from build123d import *

# Parameters (mm, degrees)
F1_DEPTH  = 31.75
F2_W      = 25.4
F2_H      = 25.4
F3_DEPTH  = 10
F4_R      = 5
F6_D      = 5.5
F8_D      = 4.2
F11_DEPTH = 5


with BuildPart() as f1:
    # F0 (on Top) → F1 (new body)
    with BuildSketch(Plane.XY):
        with BuildLine():
            Line((0, 48), (0, 0))
            Line((0, 0), (66.3673695676, 0))
            Line((66.3673695676, 0), (66.3673695676, 19.4482603496))
            ThreePointArc((66.3673695676, 19.4482603496), (67.5014803837, 21.6950829682), (69.85, 22.6))
            Line((69.85, 22.6), (100, 22.6))
            Line((100, 22.6), (100, 48))
            Line((100, 48), (0, 48))
        make_face()
    extrude(amount=F1_DEPTH)

    # F2 (on face) → F3 (cut)
    with BuildSketch(Plane(origin=(0, 0, 0), x_dir=(1, 0, 0), z_dir=(0, 0, -1))):
        with Locations((34.925, -35.3)):
            Rectangle(F2_W, F2_H)
    extrude(amount=-F3_DEPTH, mode=Mode.SUBTRACT)

    # F4
    f4_edges = [f1.edges().sort_by_distance(p)[0] for p in [
        (22.225, 22.6, 5),
        (47.625, 22.6, 5),
    ]]
    fillet(f4_edges, radius=F4_R)

    # F6 (through all)
    with Locations(Plane.XY.offset(31.75)):
        with Locations((14.1336847838, 11.3), (52.2336847838, 11.3)):
            Hole(F6_D / 2)

    # F8 (through all)
    with Locations(Plane.XY.offset(31.75)):
        with Locations((87.3, 35.3)):
            Hole(F8_D / 2)

    # F10 (on face) → F11 (cut)
    with BuildSketch(Plane(origin=(0, 0, 0), x_dir=(1, 0, 0), z_dir=(0, 0, -1))):
        with BuildLine():
            Line((17.225, -27.6), (17.225, -48))
            Line((17.225, -48), (52.625, -48))
            Line((52.625, -48), (52.625, -27.6))
            ThreePointArc((52.625, -27.6), (51.1605339059, -24.0644660941), (47.625, -22.6))
            Line((47.625, -22.6), (22.225, -22.6))
            ThreePointArc((22.225, -22.6), (18.6894660941, -24.0644660941), (17.225, -27.6))
        make_face()
    extrude(amount=-F11_DEPTH, mode=Mode.SUBTRACT)


solid = f1.part
Model file for the job. Use its own axes, mm. A direction names the side the tool comes from. Round coordinates to 2 decimals unless told otherwise and drop trailing zeros. Order: outer loops, then holes, each group sorted by start corner. A loop starts at its lowest first (then second) coordinate and runs counter-clockwise, first axis right, second up. Notation, with made-up numbers: M -36,82 L 14,82 A19 cw 14,94 Z; hole C -4,-13.5 d3. An arc over 180 degrees is marked long. Write each question's results on one line, items separated by ' | '. Start each with the question number.
(1) Saw through at B-B, the plane x = 87.3. Give the cut face in (y, z).
(2) Saw through at D-D, the plane z = 26. Give the cut face in (x, y), then the cut area to 3 significant figures.
(3) Probe probe 1 along Y at (x, z) = (87, 20); probe 2 along X at (y, z) = (44.5, 7.5) (3 decimals); probe 3 along Y at (x, z) = (85, 3.5). List the from-to ranges inside material, lowest first. Write a range as from..to.
(4) Which spindle directions (+Z, -Z, +X, -X, +Y, -Y) get a long thin tool onto all of the face, cutting with end or side? Do faces 1 (the face through (85, 22.6, 16)), 2 (the face through (16.32, 9.63, 15.65)), 3 (the face through (23.651, 24.104, 7.535)). Say none if no direction does.
(5) Drop flat-ended pins along their axis: pin 1 (9.5 mm diameter, centred on y = 5.5, z = 21, fed in from +X); pin 2 (11 mm diameter, centred on x = 47, y = 30, fed in from -Z); pin 3 (1.5 mm diameter, centred on x = 10.5, z = 4, fed in from -Y); pin 4 (3 mm diameter, centred on x = 30.5, z = 3.5, fed in from +Y). Give the stop position or say it passes through.
(6) Two-plate mould, pull along X, no slides. Class faces 4 (the face through (22.225, 38, 7)), 5 (the face through (0, 24, 16)), 6 (the face through (38, 24, 31.75)): pulls with the +X half, pulls with the -X half, needs draft (parallel to the pull), parting line crosses it, or undercut.
(7) Saw through at A-A, the plane y = 11.3. Give the cut face in (x, z).
(8) Saw through at C-C, the plane y = 35.3. Give the cut face in (x, z) (3 decimals).
Established:
1) outline: M 22.6,0 L 33.2,0 L 33.2,31.75 L 22.6,31.75 Z; M 37.4,0 L 48,0 L 48,31.75 L 37.4,31.75 Z
2) outline: M 0,0 L 66.37,0 L 66.37,19.45 A3.5 cw 69.85,22.6 L 100,22.6 L 100,48 L 0,48 Z; hole C 14.13,11.3 d5.5; hole C 52.23,11.3 d5.5; hole C 87.3,35.3 d4.2 | area: 3,980 mm^2
3) probe 1: y = 22.6..33.22, 37.38..48 | probe 2: x = 0..22.225, 47.625..100 | probe 3: y = 22.6..48
4) face 1: +Z, -Z, +X, -Y | face 2: +Z, -Z | face 3: -Z, +Y
5) pin 1: stops at x = 66.37 | pin 2: stops at z = 5 | pin 3: stops at y = 0 | pin 4: stops at y = 22.6
6) face 4: undercut | face 5: pulls with the -X half | face 6: needs draft
7) outline: M 0,0 L 11.38,0 L 11.38,31.75 L 0,31.75 Z; M 16.88,0 L 49.48,0 L 49.48,31.75 L 16.88,31.75 Z; M 54.98,0 L 66.37,0 L 66.37,31.75 L 54.98,31.75 Z
8) outline: M 0,0 L 17.225,0 L 17.225,5 L 22.225,5 L 22.225,10 L 47.625,10 L 47.625,5 L 52.625,5 L 52.625,0 L 85.2,0 L 85.2,31.75 L 0,31.75 Z; M 89.4,0 L 100,0 L 100,31.75 L 89.4,31.75 Z
